Read the model definition and answer for the solid it produces. Units are mm, in the model's axes. Face numbers are marked on the shaded views. A direction names the side the tool comes from. Coordinates: 2 decimals unless noted, no trailing zeros. Write each loop counter-clockwise with the first axis right and the second up, starting at its lowest first coordinate (ties: lowest second). Pieces come first, ordered by that corner, then holes. Notation, with made-up numbers: (-14, -28) -> (41, -28) arc R14 ccw to (41, -4) -> close; hole circle Ø3 at (-26.75, 4.5). An arc over 180 degrees is marked (long way). Return JSON: item names as keys, results as strings.
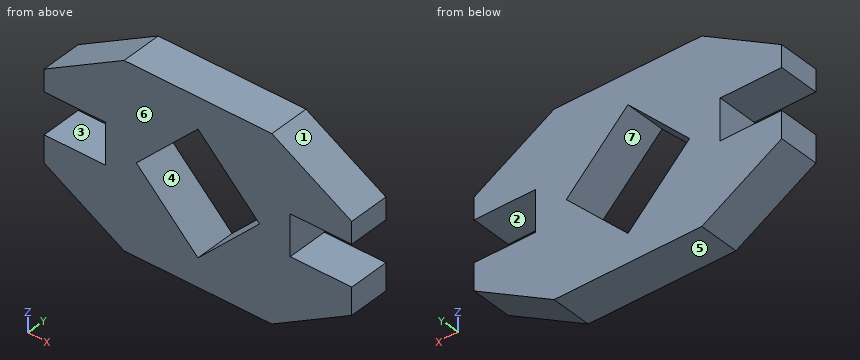
from build123d import *

# Parameters (mm, degrees)
F1_DEPTH = 25.4


with BuildPart() as f1:
    # F0 (on Front) → F1 (new body)
    with BuildSketch(Plane.XZ):
        Polygon((-37.432403, 0.733686), (0, 38.166089), (37.432403, 0.733686), (57.15, 0.733686), (57.15, 15.022763), (95.25, 15.022763), (95.25, 28.575), (45.756648, 57.15), (0, 57.15), (-45.756648, 57.15), (-95.25, 28.575), (-95.25, 15.022763), (-57.15, 15.022763), (-57.15, 0.733686), align=None)
        Polygon((57.15, 0.733686), (37.432403, 0.733686), (38.166089, 0), (0, -38.166089), (-38.166089, 0), (-37.432403, 0.733686), (-57.15, 0.733686), (-57.15, -10.377237), (-95.25, -10.377237), (-95.25, -27.107628), (-45.756648, -55.682628), (45.756648, -55.682628), (95.25, -27.107628), (95.25, -10.377237), (57.15, -10.377237), align=None)
    extrude(amount=F1_DEPTH)


solid = f1.part
1. The part is cut by section D-D (z = 40.5). Determine the outline of the cut face in (x, y).
Taken from the geometry:
{"outline": "(-74.6, -25.4) -> (74.6, -25.4) -> (74.6, 0) -> (-74.6, 0) -> close"}
2. Flat-ended cylindrical pins translate along their axes: pin 1 Ø5 at (y, z) = (-12.5, -5.5) entering from +X; pin 2 Ø4 at (x, z) = (2.5, -31.5) entering from -Y; pin 3 Ø1 at (x, z) = (47, 40.5) entering from +Y; pin 4 Ø2 at (y, z) = (-18, -30.5) entering from +X. Find the tip coordinate at first contact, or state that the pin passes through.
Taken from the geometry:
{"pin 1": "stops at x = 57.15", "pin 2": "passes through", "pin 3": "stops at y = 0", "pin 4": "stops at x = 91.11"}
3. Consider L1, parallel to X at y = -11.5, z = -5; L2, parallel to X at y = -5.5, z = -15; L3, parallel to Z at x = 80.5, y = -19. Determine where each line is inside the solid, lowest interval first.
Taken from the geometry:
{"L1": "x = -57.15 to -33.17, 33.17 to 57.15", "L2": "x = -95.25 to -23.17, 23.17 to 95.25", "L3": "z = -35.62 to -10.38, 15.02 to 37.09"}
4. A tool of negligible diameter and unlimited length cuts with its end or side. For the marked faces 1, 2, 3 and 4, from which of +Z, -Z, +X, -X, +Y, -Y can it reach the whole face along a straight path? Write none if from no direction.
Taken from the geometry:
{"face 1": "+Z, +X, +Y, -Y", "face 2": "+X, +Y, -Y", "face 3": "-X, +Y, -Y", "face 4": "+Y, -Y"}
5. The part is cut by section B-B (y = -19). Determine the outline of the cut face in (x, z) (3 decimals).
Taken from the geometry:
{"outline": "(-95.25, -27.108) -> (-45.757, -55.683) -> (45.757, -55.683) -> (95.25, -27.108) -> (95.25, -10.377) -> (57.15, -10.377) -> (57.15, 15.023) -> (95.25, 15.023) -> (95.25, 28.575) -> (45.757, 57.15) -> (-45.757, 57.15) -> (-95.25, 28.575) -> (-95.25, 15.023) -> (-57.15, 15.023) -> (-57.15, -10.377) -> (-95.25, -10.377) -> close; hole (-38.166, 0) -> (0, -38.166) -> (38.166, 0) -> (0, 38.166) -> close"}
6. For a pull along Z with two mould halves and no side action, classify the marked faces 5, 6 and 7 as +Z half, -Z half, draft (parallel to the pull), parting line (faces both ways), or undercut.
Taken from the geometry:
{"face 5": "-Z half", "face 6": "draft", "face 7": "undercut"}
7. The part is cut by section C-C (x = 71.5). Determine the outline of the cut face in (y, z).
Taken from the geometry:
{"outline": "(-25.4, -40.82) -> (0, -40.82) -> (0, -10.38) -> (-25.4, -10.38) -> close; (-25.4, 15.02) -> (0, 15.02) -> (0, 42.29) -> (-25.4, 42.29) -> close"}
8. The part is cut by section A-A (z = 21.5). Determine the outline of the cut face in (x, y), then the cut area to 3 significant figures.
Taken from the geometry:
{"outline": "(-95.25, -25.4) -> (-16.67, -25.4) -> (-16.67, 0) -> (-95.25, 0) -> close; (16.67, -25.4) -> (95.25, -25.4) -> (95.25, 0) -> (16.67, 0) -> close", "area": "3,990 mm2"}
